Here's how the part is built. I have some questions about the finished solid (model axes, mm). A direction names the side the tool comes from. Coordinates: 2 decimals unless noted, no trailing zeros. Order: outer loops, then holes, each group sorted by start corner. A loop starts at its lowest first (then second) coordinate and runs counter-clockwise, first axis right, second up.
```python
from build123d import *

# Parameters (mm, degrees)
SKETCH1_W            = 41.5
SKETCH1_H            = 51
SKETCH1_W_2          = 37.5
SKETCH1_H_2          = 47
BOSS_EXTRUDE1_DEPTH  = 8
SKETCH2_W            = 41.5
SKETCH2_H            = 51
BOSS_EXTRUDE2_DEPTH  = 2
FILLET1_R            = 4
FILLET2_R            = 3
SKETCH3_W            = 5.5
SKETCH3_H            = 20
BOSS_EXTRUDE3_DEPTH  = 6
SKETCH4_R            = 1.4
BOSS_EXTRUDE4_DEPTH  = 3.5
FILLET3_R            = 0.5
SKETCH5_W            = 6.5
SKETCH5_H            = 4
CUT_EXTRUDE1_DEPTH   = 34.835077952
SKETCH6_W            = 2
SKETCH6_H            = 10
BOSS_EXTRUDE6_DEPTH  = 6
FILLET4_R            = 3
SKETCH7_R            = 1.5
CUT_EXTRUDE2_DEPTH   = 2
SKETCH8_W            = 35
SKETCH8_H            = 1
CUT_EXTRUDE3_DEPTH   = 0.75
SKETCH9_W            = 9
SKETCH9_H            = 1
SKETCH9_W_2          = 8.5
CUT_EXTRUDE4_DEPTH   = 0.75
BOSS_EXTRUDE7_DEPTH  = 14
FILLET6_R            = 3
CUT_EXTRUDE5_DEPTH   = 42.779440692
MIRROR1_START        = 10.997748531
MIRROR1_DEPTH        = 3.002251469
MIRROR1_START_2      = -14
MIRROR1_2_DEPTH      = 2.9999999
MIRROR1_START_3      = -11.0000001
MIRROR1_3_DEPTH      = 21.997748631
MIRROR1_START_4      = -3
MIRROR1_4_DEPTH      = 10.290302021
SKETCH13_R           = 0.5
CUT_EXTRUDE6_DEPTH   = 11.5
CUT_EXTRUDE7_DEPTH   = 6
SKETCH15_W           = 4.2
SKETCH15_H           = 10.25
CUT_EXTRUDE8_DEPTH   = 42.779440772
SKETCH16_R           = 1.75
SKETCH16_R_2         = 0.5
BOSS_EXTRUDE8_DEPTH  = 3
CUT_EXTRUDE9_START   = -1
SKETCH17_W           = 37.5
SKETCH17_H           = 47
SKETCH17_R           = 1.75
SKETCH17_R_2         = 1.4
SKETCH17_W_2         = 4.2
SKETCH17_H_2         = 10.25
SKETCH17_W_3         = 6.5
SKETCH17_H_3         = 4
CUT_EXTRUDE9_DEPTH   = 1
CUT_EXTRUDE10_START  = -4.5
SKETCH18_R           = 1.4
CUT_EXTRUDE10_DEPTH  = 4.5
SKETCH19_W           = 4.2
SKETCH19_H           = 10.25
BOSS_EXTRUDE9_DEPTH  = 1
CUT_EXTRUDE11_START  = -4
SKETCH20_R           = 1.75
CUT_EXTRUDE11_DEPTH  = 4
SKETCH23_W           = 2.25
SKETCH23_H           = 5
CUT_EXTRUDE12_DEPTH  = 43.125071765
SKETCH26_W           = 2
SKETCH26_H           = 2
BOSS_EXTRUDE10_DEPTH = 9


with BuildPart() as part:
    # Sketch1 → Boss-Extrude1 (new body)
    with BuildSketch(Plane(origin=(0, 0, 0), x_dir=(1, 0, 0), z_dir=(0, 1, 0))):
        Rectangle(SKETCH1_W, SKETCH1_H)
        Rectangle(SKETCH1_W_2, SKETCH1_H_2, mode=Mode.SUBTRACT)
    extrude(amount=BOSS_EXTRUDE1_DEPTH)

    # Sketch2 → Boss-Extrude2 (add)
    with BuildSketch(Plane.XZ):
        Rectangle(SKETCH2_W, SKETCH2_H)
    extrude(amount=BOSS_EXTRUDE2_DEPTH)

    # Fillet1
    fillet1_edges = [part.edges().sort_by_distance(p)[0] for p in [
        (20.75, 3, -25.5),
        (20.75, 3, 25.5),
        (-20.75, 3, 25.5),
        (-20.75, 3, -25.5),
    ]]
    fillet(fillet1_edges, radius=FILLET1_R)

    # Fillet2
    fillet2_edges = [part.edges().sort_by_distance(p)[0] for p in [
        (-20.75, -2, 0),
        (0, -2, -25.5),
        (20.75, -2, 0),
        (0, -2, 25.5),
        (19.578427125, -2, -24.328427125),
        (19.578427125, -2, 24.328427125),
        (-19.578427125, -2, 24.328427125),
        (-19.578427125, -2, -24.328427125),
    ]]
    fillet(fillet2_edges, radius=FILLET2_R)

    # Sketch3 → Boss-Extrude3 (add)
    with BuildSketch(Plane(origin=(0, 0, 0), x_dir=(1, 0, 0), z_dir=(0, 1, 0))):
        with Locations((16, 13.5)):
            Rectangle(SKETCH3_W, SKETCH3_H)
    extrude(amount=BOSS_EXTRUDE3_DEPTH)

    # Sketch4 → Boss-Extrude4 (add)
    with BuildSketch(Plane(origin=(0, 0, 0), x_dir=(1, 0, 0), z_dir=(0, 1, 0))):
        with Locations(Location((0.245140852, 21.1, 0), (0, 0, 90))):
            Circle(SKETCH4_R)
        with Locations(Location((0.245140852, 6.1, 0), (0, 0, 90))):
            Circle(SKETCH4_R)
    extrude(amount=BOSS_EXTRUDE4_DEPTH)

    # Fillet3
    fillet3_edges = [part.edges().sort_by_distance(p)[0] for p in [
        (0.245140852, 3.5, -19.7),
        (0.245140852, 3.5, -4.7),
    ]]
    fillet(fillet3_edges, radius=FILLET3_R)

    # Sketch5 → Cut-Extrude1 (cut, through all)
    with BuildSketch(Plane(origin=(0, 0, 0), x_dir=(1, 0, 0), z_dir=(0, 1, 0))):
        with Locations((-3.5, 14.5)):
            Rectangle(SKETCH5_W, SKETCH5_H)
    extrude(amount=-CUT_EXTRUDE1_DEPTH, mode=Mode.SUBTRACT)

    # Sketch6 → Boss-Extrude6 (add)
    with BuildSketch(Plane(origin=(0, 8, 0), x_dir=(1, 0, 0), z_dir=(0, 1, 0))):
        with Locations((19.75, -0.5)):
            Rectangle(SKETCH6_W, SKETCH6_H)
    extrude(amount=BOSS_EXTRUDE6_DEPTH)

    # Fillet4
    fillet4_edges = [part.edges().sort_by_distance(p)[0] for p in [
        (19.75, 8, -4.5),
    ]]
    fillet(fillet4_edges, radius=FILLET4_R)
    fillet4_2_edges = [part.edges().sort_by_distance(p)[0] for p in [
        (19.75, 8, 5.5),
    ]]
    fillet(fillet4_2_edges, radius=FILLET4_R)
    fillet4_3_edges = [part.edges().sort_by_distance(p)[0] for p in [
        (19.75, 14, -4.5),
    ]]
    fillet(fillet4_3_edges, radius=FILLET4_R - 0.0001)  # a hair under: the kernel refuses the full size
    fillet4_4_edges = [part.edges().sort_by_distance(p)[0] for p in [
        (19.75, 14, 5.5),
    ]]
    fillet(fillet4_4_edges, radius=FILLET4_R - 0.0001)  # a hair under: the kernel refuses the full size

    # Sketch7 → Cut-Extrude2 (cut)
    with BuildSketch(Plane(origin=(20.75, 0, 0), x_dir=(0, 0, -1), z_dir=(1, 0, 0))):
        with Locations((-0.5, 8)):
            Circle(SKETCH7_R)
    extrude(amount=-CUT_EXTRUDE2_DEPTH, mode=Mode.SUBTRACT)

    # Sketch8 → Cut-Extrude3 (cut)
    with BuildSketch(Plane(origin=(-18.75, 0, 0), x_dir=(0, 0, -1), z_dir=(1, 0, 0))):
        with Locations((0.5, 6)):
            Rectangle(SKETCH8_W, SKETCH8_H)
    extrude(amount=-CUT_EXTRUDE3_DEPTH, mode=Mode.SUBTRACT)

    # Sketch9 → Cut-Extrude4 (cut)
    with BuildSketch(Plane.ZY.offset(-18.75)):
        with Locations((-11.5, 6)):
            Rectangle(SKETCH9_W, SKETCH9_H)
        with Locations((12.75, 6)):
            Rectangle(SKETCH9_W_2, SKETCH9_H)
    extrude(amount=-CUT_EXTRUDE4_DEPTH, mode=Mode.SUBTRACT)

    # Sketch10 → Boss-Extrude7 (add, symmetric)
    with BuildSketch(Plane(origin=(0, 0, 0), x_dir=(0, 0, -1), z_dir=(1, 0, 0))):
        with BuildLine():
            Line((-40.187882415, -2), (-25.5, 8))
            Line((-25.5, 8), (-25.5, 1))
            ThreePointArc((-25.5, 1), (-24.621320344, -1.121320344), (-22.5, -2))
            Line((-22.5, -2), (-40.187882415, -2))
        make_face()
    extrude(amount=BOSS_EXTRUDE7_DEPTH, both=True)

    # Fillet6
    fillet6_edges = [part.edges().sort_by_distance(p)[0] for p in [
        (0, -2, 40.187882415),
    ]]
    fillet(fillet6_edges, radius=FILLET6_R)

    # Sketch12 → Cut-Extrude5 (cut, symmetric)
    with BuildSketch(Plane(origin=(0, 0, 0), x_dir=(1, 0, 0), z_dir=(0, 1, 0))):
        with BuildLine():
            ThreePointArc((-10, -33.450846993), (-10.0925407, -29.937641684), (-11, -26.542396046))
            ThreePointArc((-11, -26.542396046), (-0.001557097, -28.220686258), (10.997748531, -26.548059567))
            ThreePointArc((10.997748531, -26.548059567), (10.092104456, -29.940657614), (10, -33.450846993))
            ThreePointArc((10, -33.450846993), (0, -35.763467262), (-10, -33.450846993))
        make_face()
    extrude(amount=CUT_EXTRUDE5_DEPTH, both=True, mode=Mode.SUBTRACT)

    # Mirror1: read off the stored shape, not the designer's step
    # Mirror1 outline → Mirror1 (add)
    with BuildSketch(Plane.YZ.offset(MIRROR1_START)):
        with BuildLine():
            ThreePointArc((1, -25.5), (-1.121320344, -24.621320344), (-2, -22.5))
            Line((-2, -22.5), (-2, -30.450846993))
            ThreePointArc((-2, -30.450846993), (0.116669534, -33.31785367), (3.479818192, -32.139189888))
            Line((3.479818192, -32.139189888), (8, -25.5))
            Line((8, -25.5), (1, -25.5))
        make_face()
    extrude(amount=MIRROR1_DEPTH)

    # Mirror1 2 outline → Mirror1 2 (add)
    with BuildSketch(Plane.YZ.offset(MIRROR1_START_2)):
        with BuildLine():
            ThreePointArc((1, -25.5), (-1.121320344, -24.621320344), (-2, -22.5))
            Line((-2, -22.5), (-2, -30.450846993))
            ThreePointArc((-2, -30.450846993), (0.116669534, -33.31785367), (3.479818192, -32.139189888))
            Line((3.479818192, -32.139189888), (8, -25.5))
            Line((8, -25.5), (1, -25.5))
        make_face()
    extrude(amount=MIRROR1_2_DEPTH)

    # Mirror1 3 outline → Mirror1 3 (add)
    with BuildSketch(Plane.YZ.offset(MIRROR1_START_3)):
        with BuildLine():
            ThreePointArc((1.000000002, -25.5), (-1.121320344, -24.621320344), (-2, -22.499999998))
            Line((-2, -22.499999998), (-2, -30.450846993))
            ThreePointArc((-2, -30.450846993), (0.116669534, -33.31785367), (3.479818192, -32.139189888))
            Line((3.479818192, -32.139189888), (8, -25.5))
            Line((8, -25.5), (1.000000002, -25.5))
        make_face()
    extrude(amount=MIRROR1_3_DEPTH)

    # Mirror1 4 outline → Mirror1 4 (cut)
    with BuildSketch(Plane(origin=(0, 0, 0), x_dir=(1, 0, 0), z_dir=(0, 1, 0)).offset(MIRROR1_START_4)):
        with BuildLine():
            ThreePointArc((-11, 26.542396046), (-0.001557097, 28.220686258), (10.997748531, 26.548059567))
            ThreePointArc((10.997748531, 26.548059567), (10.092086007, 29.940785259), (10.000023464, 33.451103865))
            Line((10.000023464, 33.451103865), (10.141518844, 35))
            Line((10.141518844, 35), (-10.141519787, 35))
            Line((-10.141519787, 35), (-10.000024287, 33.451112878))
            ThreePointArc((-10.000024287, 33.451112878), (-10.092521576, 29.937773803), (-11, 26.542396046))
        make_face()
    extrude(amount=MIRROR1_4_DEPTH, mode=Mode.SUBTRACT)

    # Sketch13 → Cut-Extrude6 (cut, symmetric)
    with BuildSketch(Plane(origin=(0, 0, 0), x_dir=(0, 0, -1), z_dir=(1, 0, 0))):
        with Locations(Location((-30.5, 1, 0), (0, 0, 180))):
            Circle(SKETCH13_R)
    cut_extrude6 = extrude(amount=CUT_EXTRUDE6_DEPTH, both=True, mode=Mode.SUBTRACT)

    # Mirror2: Cut-Extrude6 across plane
    add(cut_extrude6.mirror(Plane.XY), mode=Mode.SUBTRACT)

    # Sketch14 → Cut-Extrude7 (cut)
    with BuildSketch(Plane(origin=(0, 6, 0), x_dir=(1, 0, 0), z_dir=(0, 1, 0))):
        Polygon((18.75, 23.5), (13.25, 23.5), (13.25, 3.5), (18.75, 3.5), (18.75, 7), (18.75, 16), align=None)
    extrude(amount=-CUT_EXTRUDE7_DEPTH, mode=Mode.SUBTRACT)

    # Sketch15 → Cut-Extrude8 (cut, through all)
    with BuildSketch(Plane(origin=(0, 0, 0), x_dir=(1, 0, 0), z_dir=(0, 1, 0))):
        with Locations((14.15, 13.375)):
            Rectangle(SKETCH15_W, SKETCH15_H)
    extrude(amount=-CUT_EXTRUDE8_DEPTH, mode=Mode.SUBTRACT)

    # Sketch16 → Boss-Extrude8 (add)
    with BuildSketch(Plane(origin=(0, 0, 0), x_dir=(1, 0, 0), z_dir=(0, 1, 0))):
        with Locations(Location((-16.25, 19.5, 0), (0, 0, 90))):
            Circle(SKETCH16_R)
        with Locations(Location((-16.25, 19.5, 0), (0, 0, 270))):
            Circle(SKETCH16_R_2, mode=Mode.SUBTRACT)
    extrude(amount=BOSS_EXTRUDE8_DEPTH)

    # Sketch17 → Cut-Extrude9 (cut)
    with BuildSketch(Plane(origin=(0, 0, 0), x_dir=(1, 0, 0), z_dir=(0, 1, 0)).offset(CUT_EXTRUDE9_START)):
        Rectangle(SKETCH17_W, SKETCH17_H)
        with Locations(Location((-16.25, 19.5, 0), (0, 0, 270))):
            Circle(SKETCH17_R, mode=Mode.SUBTRACT)
        with Locations(Location((0.245140852, 21.1, 0), (0, 0, 270))):
            Circle(SKETCH17_R_2, mode=Mode.SUBTRACT)
        with Locations(Location((0.245140852, 6.1, 0), (0, 0, 270))):
            Circle(SKETCH17_R_2, mode=Mode.SUBTRACT)
        with Locations((14.15, 13.375)):
            Rectangle(SKETCH17_W_2, SKETCH17_H_2, mode=Mode.SUBTRACT)
        with Locations((-3.5, 14.5)):
            Rectangle(SKETCH17_W_3, SKETCH17_H_3, mode=Mode.SUBTRACT)
    extrude(amount=CUT_EXTRUDE9_DEPTH, mode=Mode.SUBTRACT)

    # Sketch18 → Cut-Extrude10 (cut)
    with BuildSketch(Plane(origin=(0, 3.5, 0), x_dir=(1, 0, 0), z_dir=(0, 1, 0)).offset(CUT_EXTRUDE10_START)):
        with Locations((0.245140852, 21.1)):
            Circle(SKETCH18_R)
        with Locations((0.245140852, 6.1)):
            Circle(SKETCH18_R)
    extrude(amount=CUT_EXTRUDE10_DEPTH, mode=Mode.SUBTRACT)

    # Sketch19 → Boss-Extrude9 (add)
    with BuildSketch(Plane.XZ.offset(2)):
        with Locations((14.15, -13.375)):
            Rectangle(SKETCH19_W, SKETCH19_H)
    extrude(amount=-BOSS_EXTRUDE9_DEPTH)

    # Sketch20 → Cut-Extrude11 (cut)
    with BuildSketch(Plane(origin=(0, 3, 0), x_dir=(1, 0, 0), z_dir=(0, 1, 0)).offset(CUT_EXTRUDE11_START)):
        with Locations((-16.25, 19.5)):
            Circle(SKETCH20_R)
    extrude(amount=CUT_EXTRUDE11_DEPTH, mode=Mode.SUBTRACT)

    # Sketch23 → Cut-Extrude12 (cut, through all)
    with BuildSketch(Plane(origin=(0, -1, 0), x_dir=(1, 0, 0), z_dir=(0, 1, 0))):
        with Locations((-16.375, 14)):
            Rectangle(SKETCH23_W, SKETCH23_H)
    extrude(amount=-CUT_EXTRUDE12_DEPTH, mode=Mode.SUBTRACT)

    # Sketch26 → Boss-Extrude10 (add)
    with BuildSketch(Plane(origin=(0, -1, 0), x_dir=(1, 0, 0), z_dir=(0, 1, 0))):
        with Locations((-2.25, 22.5)):
            Rectangle(SKETCH26_W, SKETCH26_H)
        with Locations((15.75, 22.5)):
            Rectangle(SKETCH26_W, SKETCH26_H)
    extrude(amount=BOSS_EXTRUDE10_DEPTH)


solid = part.part
```
Q1. I need wall thicknesses on L1, parallel to X at y = 3, z = -6; L2, parallel to Y at x = 0, z = -20.5; L3, parallel to Z at x = 9, y = 0.25. Which ranges of each line are inside material? Lowest first, please.
Q2. Will these pins go through, and if not, where does the flat tip stop? pin 1 (1.1 mm diameter, centred on y = -1.5, z = -14, fed in from -X); pin 2 (0.8 mm diameter, centred on y = -1.5, z = -15, fed in from -X); pin 3 (3 mm diameter, centred on y = 3, z = 26.5, fed in from -X); pin 4 (4 mm diameter, centred on y = 8, z = 0.5, fed in from +X).
Q3. For faces 1 (the cylindrical face through (-15.36, -1.1, 24.64)), 2 (the flat face through (15, 5, -25.5)), 3 (the flat face through (-11, 3, -23.5)), 4 (the cylindrical face through (19.89, -1.1, -0.3)), which set-ups out of +Z, -Z, +X, -X, +Y, -Y let a thin tool reach every point of the face, with its end or its side?
Q4. If we section it at A-A on z = 0.5: Write out the boundary of the cut face in (x, y).
Q5. If we section it at B-B on y = 12.75: Write out the boundary of the cut face in (x, z), then the cut area to 3 significant figures.
Q6. We'd pull the mould along X, two halves only. Please class faces 5 (the cylindrical face through (11.997, 0.168, 33.333)), 6 (the cylindrical face through (-10.215, 1.678, 29.215)), 7 (the flat face through (-14, 2, 29)): pulls with the +X half, pulls with the -X half, needs draft (parallel to the pull), parting line crosses it, or undercut.
Reply:
1. L1: x = -20.75 to -18.75, 18.75 to 20.75
1. L2: y = -2 to -1
1. L3: z = -27.11 to -23.5, 23.5 to 27.11
2. pin 1: stops at x = -20.03
2. pin 2: stops at x = -19.89
2. pin 3: stops at x = -18.69
2. pin 4: stops at x = 20.75
3. face 1: +Z, -X, -Y
3. face 2: -Z, +X, +Y, -Y
3. face 3: +Y
3. face 4: +Z, -Z, +X, -Y
4. outline: (-20.75, 1) arc R3 ccw to (-17.75, -2) - (17.75, -2) arc R3 ccw to (20.75, 1) - (20.75, 6.5) - (18.75, 6.5) - (18.75, -1) - (-18.75, -1) - (-18.75, 5.5) - (-19.5, 5.5) - (-19.5, 6.5) - (-18.75, 6.5) - (-18.75, 8) - (-20.75, 8) - close; (18.75, 9.5) - (20.75, 9.5) - (20.75, 14) - (18.75, 14) - close
5. outline: (18.75, -3.94) - (20.75, -3.94) - (20.75, 4.94) - (18.75, 4.94) - close
5. area: 17.7 mm2
6. face 5: needs draft
6. face 6: undercut
6. face 7: pulls with the -X half
